For this review, use the dimensioned drawing (mm, ordinates from the lowest corner) and the shaded views. A direction names the side the tool comes from. Coordinates: 2 decimals unless noted, no trailing zeros. Loops run counter-clockwise (first coordinate to the right, second up) from the corner with the lowest first, then second, coordinate; pieces in that order, holes last. Notation, with made-up numbers: (25.25, 57) -> (36.25, 57) arc R9 cw to (36.25, 61) -> close; hole circle Ø4 at (-29, 39). An arc over 180 degrees is marked (long way). Use one line per item in the form item = value. Start each with the question number.
1. Wall thickness on line 1 (X direction, y = 362.5, z = 524.5); line 2 (Z direction, x = 96.5, y = 27); line 3 (Z direction, x = 706, y = 218): over which ranges is each line inside the solid? List them lowest first. Write a range as from..to.
2. Consider section C-C (y = 361). State the section outline as (x, z) points.
3. Consider section A-A (x = 57). State the section outline as (y, z) points.
4. Consider section D-D (x = 807.5). State the section outline as (y, z) points, then the cut area to 3 significant figures.
5. Machinability: for the marked faces 1 and 2, which of the approach directions +Z, -Z, +X, -X, +Y, -Y give a long, thin tool a straight path to every point of the face, cutting with its end or side? Answer none if there is none.
6. The part is to be moulded in two halves that separate along Z. For the marked faces 3, 4 and 5, say which applies: released by +Z, released by -Z, zero draft, split by the parting line, or undercut.
7. For pin 1 (4 mm diameter, centred on x = 527.5, y = 120.5, fed in from +Z), flat-tipped, find the tip position at first contact; note if it passes through.
8. Consider section B-B (z = 625). State the section outline as (x, y) points, then the cut area to 3 significant figures.
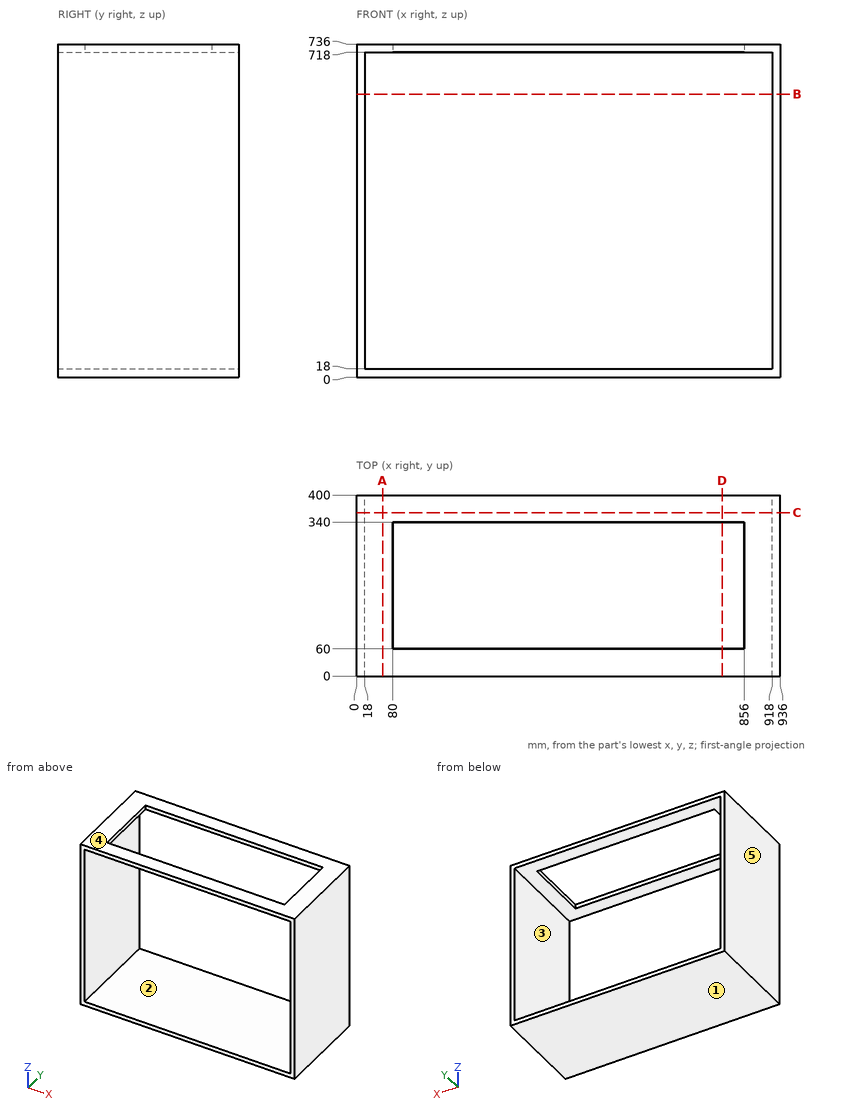
Geometry check:
q1.line_1 = 0..18, 918..936
q1.line_2 = 0..18, 718..736
q1.line_3 = 0..18
q2.outline = (0, 0) -> (936, 0) -> (936, 736) -> (0, 736) -> close; hole (18, 18) -> (918, 18) -> (918, 718) -> (18, 718) -> close
q3.outline = (0, 0) -> (400, 0) -> (400, 18) -> (0, 18) -> close; (0, 718) -> (400, 718) -> (400, 736) -> (0, 736) -> close
q4.outline = (0, 0) -> (400, 0) -> (400, 18) -> (0, 18) -> close; (0, 718) -> (60, 718) -> (60, 736) -> (0, 736) -> close; (340, 718) -> (400, 718) -> (400, 736) -> (340, 736) -> close
q4.area = 9,360 mm²
q5.face_1 = -Z, +X, -X, +Y, -Y
q5.face_2 = +Y, -Y
q6.face_3 = undercut
q6.face_4 = released by +Z
q6.face_5 = zero draft
q7.pin_1 = 18
q8.outline = (0, 0) -> (18, 0) -> (18, 400) -> (0, 400) -> close; (918, 0) -> (936, 0) -> (936, 400) -> (918, 400) -> close
q8.area = 14,400 mm²
